Can you work these out from the model? Positions are in its coordinate system, mm. A direction names the side the tool comes from. Give positions to 0.01 mm unless a question says otherwise; leave off trailing zeros. Order: outer loops, then holes, each group sorted by start corner. A loop starts at its lowest first (then second) coordinate and runs counter-clockwise, first axis right, second up. Notation, with made-up numbers: (-24.75, 7.25) - (10.25, 7.25) arc R21 ccw to (10.25, 20.25) - close; hole circle Ø11 at (11, -25). An arc over 180 degrees is marked (long way). Return JSON: item names as keys, results as strings.
```python
from build123d import *

# Parameters (mm, degrees)
F0_W      = 66.675
F0_H      = 142.24
F1_DEPTH  = 10.16
F2_W      = 66.675
F2_H      = 142.494
F3_DEPTH  = 8.382
F4_R      = 9.525
F5_W      = 47.625
F5_H      = 5.08
F5_W_2    = 5.08
F5_H_2    = 11.1125
F5_H_3    = 26.9875
F6_DEPTH  = 7.874
F7_W      = 27.94
F7_H      = 17.4625
F8_DEPTH  = 2.286
F9_R      = 2.54
F10_W     = 5.08
F10_H     = 26.9875
F11_DEPTH = 1.27
F12_W     = 5.08
F12_H     = 11.1125
F13_DEPTH = 1.27
F14_W     = 47.625
F14_H     = 5.08
F15_DEPTH = 0.762


with BuildPart() as f1:
    # F0 (on Top) → F1 (new body)
    with BuildSketch(Plane.XY):
        Polygon((-38.4175, -76.2), (-33.3375, -76.2), (38.4175, -76.2), (38.4175, 76.2), (-38.4175, 76.2), align=None)
        Rectangle(F0_W, F0_H, mode=Mode.SUBTRACT)
        Rectangle(F0_W, F0_H)
    extrude(amount=F1_DEPTH)

    # F2 (on face) → F3 (cut)
    with BuildSketch(Plane.XY.offset(10.16)):
        with Locations((0, 0.127)):
            Rectangle(F2_W, F2_H)
    extrude(amount=-F3_DEPTH, mode=Mode.SUBTRACT)

    # F4
    f4_edges = [f1.edges().sort_by_distance(p)[0] for p in [
        (-38.4175, 76.2, 5.08),
        (-38.4175, -76.2, 5.08),
        (-33.3375, 71.374, 5.969),
        (-33.3375, -71.12, 5.969),
        (33.3375, -71.12, 5.969),
        (38.4175, -76.2, 5.08),
        (38.4175, 76.2, 5.08),
        (33.3375, 71.374, 5.969),
    ]]
    fillet(f4_edges, radius=F4_R)

    # F5 (on face) → F6 (cut)
    with BuildSketch(Plane.XY.offset(10.16)):
        with Locations((0, -73.66)):
            Rectangle(F5_W, F5_H)
        with Locations((35.8775, 24.60625)):
            Rectangle(F5_W_2, F5_H_2)
        with Locations((-35.8775, 40.48125)):
            Rectangle(F5_W_2, F5_H_3)
    extrude(amount=-F6_DEPTH, mode=Mode.SUBTRACT)

    # F7 (on face) → F8 (cut)
    with BuildSketch(Plane(origin=(0, 0, 0), x_dir=(1, 0, 0), z_dir=(0, 0, -1))):
        with Locations((5.3975, -51.59375)):
            Rectangle(F7_W, F7_H)
    extrude(amount=-F8_DEPTH, mode=Mode.SUBTRACT)

    # F9
    f9_edges = [f1.edges().sort_by_distance(p)[0] for p in [
        (19.3675, 60.325, 0.889),
        (-8.5725, 60.325, 0.889),
        (-8.5725, 42.8625, 0.889),
        (19.3675, 42.8625, 0.889),
    ]]
    fillet(f9_edges, radius=F9_R)

    # F10 (on face) → F11 (join)
    with BuildSketch(Plane.XY.offset(10.16)):
        with Locations((-35.8775, 40.48125)):
            Rectangle(F10_W, F10_H)
    extrude(amount=-F11_DEPTH)

    # F12 (on face) → F13 (join)
    with BuildSketch(Plane.XY.offset(10.16)):
        with Locations((35.8775, 24.60625)):
            Rectangle(F12_W, F12_H)
    extrude(amount=-F13_DEPTH)

    # F14 (on face) → F15 (join)
    with BuildSketch(Plane.XY.offset(10.16)):
        with Locations((0, -73.66)):
            Rectangle(F14_W, F14_H)
    extrude(amount=-F15_DEPTH)


solid = f1.part
```
1. Suppose I cut it at D-D (x = 15). List the corners of the cut face in (y, z) for me (1 decimal).
Checks:
{"outline": "(-76.2, 0) - (42.9, 0) - (42.9, 1.8) - (-71.1, 1.8) - (-71.1, 2.3) - (-76.2, 2.3) - close; (-76.2, 9.4) - (-71.1, 9.4) - (-71.1, 10.2) - (-76.2, 10.2) - close; (60.3, 0) - (76.2, 0) - (76.2, 10.2) - (71.4, 10.2) - (71.4, 1.8) - (60.3, 1.8) - close"}
2. Suppose I cut it at B-B (z = 4.75). State how many separate pieces and enclosed holes the cut face has, plus the area to 3 significant figures.
Checks:
{"separate pieces": "3", "enclosed holes": "0", "area": "1,770 mm^2"}
3. For pin 1 Ø4 at (x, y) = (0.5, -72.5) entering from -Z; pin 2 Ø4 at (x, z) = (36.5, 5) entering from -Y; pin 3 Ø1.5 at (y, z) = (-74, 7) entering from -X; pin 4 Ø1.5 at (x, z) = (-35.5, 5) entering from +Y, each with a flat end and sliding along its axis, tell me the tip position at first contact or that it passes through.
Checks:
{"pin 1": "z = 0", "pin 2": "y = -74.37", "pin 3": "x = -35.78", "pin 4": "y = 74.19"}
4. If I drill on L1, parallel to X at y = -56.5, z = 9.75; L2, parallel to Y at x = 3.5, z = 1.5 (1 decimal); L3, parallel to Z at x = -9, y = -57.5, over which ranges is the centre line in solid material (lowest first)? Write a range as [from, to].
Checks:
{"L1": "[-38.42, -33.34], [33.34, 38.42]", "L2": "[-76.2, 42.9], [60.3, 76.2]", "L3": "[0, 1.78]"}
5. On a 3-axis mill with a long thin cutter (end or side, diameter ignored), from which of +Z, -Z, +X, -X, +Y, -Y can I reach the whole of each face in a straight line? I mean faces 1 (the face through (-30.47, 68.66, 5.91)), 2 (the face through (-35.553, -73.484, 5.151)), 3 (the face through (-36, 26.988, 6)), 4 (the face through (0, -74, 2.286)), 5 (the face through (-36, 41, 2.286)). Say none if no direction works.
Checks:
{"face 1": "+Z", "face 2": "+Z, -Z, -X, -Y", "face 3": "+X, -X", "face 4": "-Y", "face 5": "-X"}
6. Suppose I cut it at C-C (x = -12.5). List the corners of the cut face in (y, z) for me.
Checks:
{"outline": "(-76.2, 0) - (76.2, 0) - (76.2, 10.16) - (71.37, 10.16) - (71.37, 1.78) - (-71.12, 1.78) - (-71.12, 2.29) - (-76.2, 2.29) - close; (-76.2, 9.4) - (-71.12, 9.4) - (-71.12, 10.16) - (-76.2, 10.16) - close"}
7. Suppose I cut it at A-A (y = 25.5). List the corners of the cut face in (x, z) for me.
Checks:
{"outline": "(-38.42, 0) - (38.42, 0) - (38.42, 2.29) - (33.34, 2.29) - (33.34, 1.78) - (-33.34, 1.78) - (-33.34, 10.16) - (-38.42, 10.16) - close; (33.34, 8.89) - (38.42, 8.89) - (38.42, 10.16) - (33.34, 10.16) - close"}
8. Thinking about a two-plate mould opening in Z: for faces 6 (the face through (0, 1, 1.778)), 7 (the face through (-30.473, -68.404, 5.91)), 8 (the face through (36, 25, 8.89)), 9 (the face through (0, -74, 9.398)), which applies, +Z half, -Z half, draft (parallel to the pull), parting line (faces both ways), or undercut?
Checks:
{"face 6": "+Z half", "face 7": "draft", "face 8": "undercut", "face 9": "undercut"}
